from build123d import *

# Parameters (mm, degrees)
F1_DEPTH = 35.75


# Not quite as in the source:
# - a feature names something its author has since deleted; it is built from what else it names


with BuildPart() as f1:
    # F0 (on Top) → F1 (new body)
    with BuildSketch(Plane.XY):
        with BuildLine():
            ThreePointArc((-0.5, 15.0505102572), (-0.251272405, 15.0126596175), (0, 15))
            Line((0, 15), (0, 16))
            ThreePointArc((0, 16), (-1.0606601718, 16.4393398282), (-1.5, 17.5))
            Line((-1.5, 17.5), (-2.5, 17.5))
            ThreePointArc((-2.5, 17.5), (-1.9364916731, 15.9188611699), (-0.5, 15.0505102572))
        make_face()
        with BuildLine():
            Line((0, 16), (0, 15))
            ThreePointArc((0, 15), (0.251272405, 15.0126596175), (0.5, 15.0505102572))
            ThreePointArc((0.5, 15.0505102572), (1.9364916731, 15.9188611699), (2.5, 17.5))
            Line((2.5, 17.5), (1.5, 17.5))
            ThreePointArc((1.5, 17.5), (1.0606601718, 16.4393398282), (0, 16))
        make_face()
        with BuildLine():
            ThreePointArc((0.5, 15.0505102572), (0.251272405, 15.0126596175), (0, 15))
            ThreePointArc((0, 15), (-0.251272405, 15.0126596175), (-0.5, 15.0505102572))
            Line((-0.5, 15.0505102572), (-0.5, -15.0505102572))
            ThreePointArc((-0.5, -15.0505102572), (0, -15), (0.5, -15.0505102572))
            Line((0.5, -15.0505102572), (0.5, 15.0505102572))
        make_face()
        with BuildLine():
            ThreePointArc((0.5, -15.0505102572), (0, -15), (-0.5, -15.0505102572))
            ThreePointArc((-0.5, -15.0505102572), (-1.9364916731, -15.9188611699), (-2.5, -17.5))
            Line((-2.5, -17.5), (-1.5, -17.5))
            ThreePointArc((-1.5, -17.5), (0, -16), (1.5, -17.5))
            Line((1.5, -17.5), (2.5, -17.5))
            ThreePointArc((2.5, -17.5), (1.9364916731, -15.9188611699), (0.5, -15.0505102572))
        make_face()
    extrude(amount=F1_DEPTH)


solid = f1.part
The listing builds one solid part. Answer for the finished solid, in the listing's coordinates (mm). A direction names the side the tool comes from. Round coordinates to 2 decimals unless told otherwise and drop trailing zeros. Write each loop counter-clockwise with the first axis right and the second up, starting at its lowest first coordinate (ties: lowest second). Pieces come first, ordered by that corner, then holes. Notation, with made-up numbers: M -12,33.5 L 16,33.5 A11 cw 16,43.5 Z; hole C -35,60.25 d1. An arc over 180 degrees is marked long. Write each question's results on one line, items separated by ' | '. Start each with the question number.
Item 1: Flat-ended cylindrical pins translate along their axes: pin 1 Ø2 at (x, y) = (2, 14) entering from -Z; pin 2 Ø12 at (y, z) = (0, 18.5) entering from +X; pin 3 Ø6 at (y, z) = (-1, 6) entering from -X. Find the tip coordinate at first contact, or state that the pin passes through.
Item 2: A cutting plane is placed at C-C on y = 15.5. Write down the section's boundary in (x, z), and give its area (3 significant figures).
Item 3: A cutting plane is placed at B-B on z = 23. Write down the section's boundary in (x, y), and give its area (3 significant figures).
Item 4: A cutting plane is placed at A-A on x = 1. Write down the section's boundary in (y, z), and give its area (3 significant figures).
Item 5: For faces 4 (the face through (0, -1, 35.75)), 5 (the face through (2, 16, 18)), 6 (the face through (-2, 16, 18)), determine the directions among +Z, -Z, +X, -X, +Y, -Y from which every point of the face is accessible in a straight line to the end or side of a thin tool.
Item 6: For a pull along X with two mould halves and no side action, classify faces 1 (the face through (-2, -16, 18)), 2 (the face through (0, -1, 0)), 3 (the face through (0, -16, 18)) as pulls with the +X half, pulls with the -X half, needs draft (parallel to the pull), parting line crosses it, or undercut.
Item 7: Straight lines are drawn through the part: L1, parallel to X at y = -4, z = 26; L2, parallel to X at y = -15.5, z = 5; L3, parallel to Y at x = 0.9, z = 5. For each, find the intervals that lie inside material, in ascending order. Write a range as [from, to].
Check sheet entries:
1) pin 1: through | pin 2: x = 0.5 | pin 3: x = -0.5
2) outline: M -1.5,0 L 1.5,0 L 1.5,35.75 L -1.5,35.75 Z | area: 107 mm²
3) outline: M -2.5,-17.5 L -1.5,-17.5 A1.5 cw 1.5,-17.5 L 2.5,-17.5 A2.5 ccw 0.5,-15.05 L 0.5,15.05 A2.5 ccw 2.5,17.5 L 1.5,17.5 A1.5 cw -1.5,17.5 L -2.5,17.5 A2.5 ccw -0.5,15.05 L -0.5,-15.05 A2.5 ccw Z | area: 42.6 mm²
4) outline: M -16.38,0 L -15.21,0 L -15.21,35.75 L -16.38,35.75 Z; M 15.21,0 L 16.38,0 L 16.38,35.75 L 15.21,35.75 Z | area: 83.9 mm²
5) face 4: +Z, +X, -X, +Y, -Y | face 5: +Z, -Z, +X | face 6: +Z, -Z, -X
6) face 1: pulls with the -X half | face 2: needs draft | face 3: undercut
7) L1: [-0.5, 0.5] | L2: [-1.5, 1.5] | L3: [-16.3, -15.17], [15.17, 16.3]
